from build123d import *

# Parameters (mm, degrees)
SKETCH1_W           = 90
SKETCH1_H           = 155.172413794
SKETCH1_R           = 1.655172414
BOSS_EXTRUDE1_DEPTH = 3
CUT_EXTRUDE1_DEPTH  = 90.741960646
CHAMFER1_SIZE       = 1
CHAMFER2_SIZE       = 1


with BuildPart() as part:
    # Sketch1 → Boss-Extrude1 (new body)
    with BuildSketch(Plane(origin=(0, 0, 0), x_dir=(1, 0, 0), z_dir=(0, 1, 0))):
        Rectangle(SKETCH1_W, SKETCH1_H)
        with Locations(Location((38.5, -70, 0), (0, 0, 270))):
            Circle(SKETCH1_R, mode=Mode.SUBTRACT)
        with Locations(Location((-38.5, -70, 0), (0, 0, 270))):
            Circle(SKETCH1_R, mode=Mode.SUBTRACT)
        with Locations(Location((38.5, 70, 0), (0, 0, 270))):
            Circle(SKETCH1_R, mode=Mode.SUBTRACT)
        with Locations(Location((-38.5, 70, 0), (0, 0, 270))):
            Circle(SKETCH1_R, mode=Mode.SUBTRACT)
    extrude(amount=BOSS_EXTRUDE1_DEPTH)

    # Sketch2 → Cut-Extrude1 (cut, through all)
    with BuildSketch(Plane(origin=(0, 3, 0), x_dir=(1, 0, 0), z_dir=(0, 1, 0))):
        with BuildLine():
            ThreePointArc((-39.9, 46.5), (-42.63137085, 47.63137085), (-41.5, 44.9))
            Line((-41.5, 44.9), (-41.5, 46.5))
            Line((-41.5, 46.5), (-39.9, 46.5))
        make_face()
        with BuildLine():
            Line((-41.5, 46.5), (-41.5, 44.9))
            ThreePointArc((-41.5, 44.9), (-40.36862915, 45.36862915), (-39.9, 46.5))
            Line((-39.9, 46.5), (-41.5, 46.5))
        make_face()
        with BuildLine():
            ThreePointArc((39.9, 46.5), (40.36862915, 45.36862915), (41.5, 44.9))
            Line((41.5, 44.9), (41.5, 46.5))
            Line((41.5, 46.5), (39.9, 46.5))
        make_face()
        with BuildLine():
            Line((41.5, 46.5), (41.5, 44.9))
            ThreePointArc((41.5, 44.9), (42.63137085, 45.36862915), (43.1, 46.5))
            ThreePointArc((43.1, 46.5), (41.5, 48.1), (39.9, 46.5))
            Line((39.9, 46.5), (41.5, 46.5))
        make_face()
        with BuildLine():
            ThreePointArc((41.5, -44.9), (40.36862915, -45.36862915), (39.9, -46.5))
            Line((39.9, -46.5), (41.5, -46.5))
            Line((41.5, -46.5), (41.5, -44.9))
        make_face()
        with BuildLine():
            Line((41.5, -46.5), (39.9, -46.5))
            ThreePointArc((39.9, -46.5), (41.5, -48.1), (43.1, -46.5))
            ThreePointArc((43.1, -46.5), (42.63137085, -45.36862915), (41.5, -44.9))
            Line((41.5, -44.9), (41.5, -46.5))
        make_face()
        with BuildLine():
            Line((-41.5, -44.9), (-41.5, -46.5))
            Line((-41.5, -46.5), (-39.9, -46.5))
            ThreePointArc((-39.9, -46.5), (-40.36862915, -45.36862915), (-41.5, -44.9))
        make_face()
        with BuildLine():
            Line((-39.9, -46.5), (-41.5, -46.5))
            Line((-41.5, -46.5), (-41.5, -44.9))
            ThreePointArc((-41.5, -44.9), (-42.63137085, -47.63137085), (-39.9, -46.5))
        make_face()
    extrude(amount=-CUT_EXTRUDE1_DEPTH, mode=Mode.SUBTRACT)

    # Chamfer1
    chamfer1_edges = [part.edges().sort_by_distance(p)[0] for p in [
        (0, 3, 77.586206897),
        (0, 3, -77.586206897),
    ]]
    chamfer(chamfer1_edges, length=CHAMFER1_SIZE)

    # Chamfer2
    chamfer2_edges = [part.edges().sort_by_distance(p)[0] for p in [
        (45, 3, 0),
        (-45, 3, 0),
    ]]
    chamfer(chamfer2_edges, length=CHAMFER2_SIZE)


solid = part.part
Work out the finished part from the listing and answer in its coordinate system (mm). Give positions to 0.01 mm unless a question says otherwise; leave off trailing zeros. Order: outer loops, then holes, each group sorted by start corner. A loop starts at its lowest first (then second) coordinate and runs counter-clockwise, first axis right, second up. Notation, with made-up numbers: M -34.75,-4 L -5.75,-4 A23 cw -5.75,24 Z; hole C 38.25,66.5 d5. An arc over 180 degrees is marked long. Return JSON: item names as keys, results as strings.
Q1. Find section A-A, the plane z = -70. Write down the section's boundary in (x, y), and give its area (3 significant figures).
Answer below:
{"outline": "M -45,0 L -40.16,0 L -40.16,3 L -44,3 L -45,2 Z; M -36.84,0 L 36.84,0 L 36.84,3 L -36.84,3 Z; M 40.16,0 L 45,0 L 45,2 L 44,3 L 40.16,3 Z", "area": "249 mm^2"}
Q2. The mould has two halves that part along X. Classify faces 1 (the face through (-1, 3, -1)), 2 (the face through (-39.13, 1.48, 71.53)): pulls with the +X half, pulls with the -X half, needs draft (parallel to the pull), parting line crosses it, or undercut.
Answer below:
{"face 1": "needs draft", "face 2": "undercut"}
Q3. Find the intervals of material crossed by line 1 along X through (y, z) = (0.95, 46.5); line 2 along X through (y, z) = (0.75, -70); line 3 along Z through (x, y) = (-41.5, 1.2), in increasing order. Write a range as [from, to].
Answer below:
{"line 1": "x = [-45, -43.1], [-39.9, 39.9], [43.1, 45]", "line 2": "x = [-45, -40.16], [-36.84, 36.84], [40.16, 45]", "line 3": "z = [-77.59, -48.1], [-44.9, 44.9], [48.1, 77.59]"}
Q4. This flat-tipped pin is pushed along its axis until it touches: pin 1 (2 mm diameter, centred on x = -38.5, z = -70, fed in from -Y). Where does it stop, or does it pass through?
Answer below:
{"pin 1": "passes through"}
